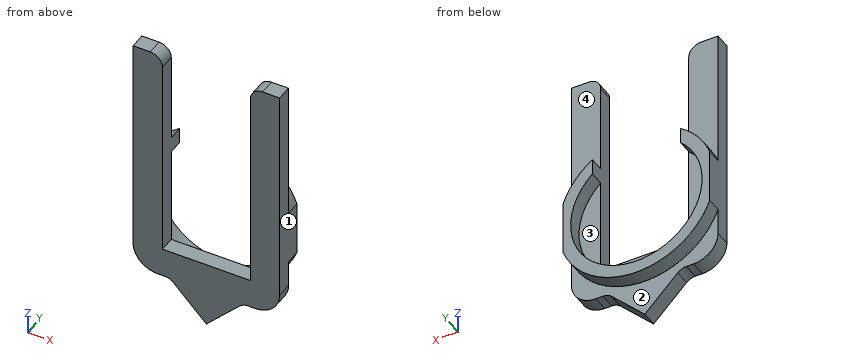
```python
from build123d import *

# Parameters (mm, degrees)
BOSS_EXTRUDE1_DEPTH = 3.2
BOSS_EXTRUDE2_DEPTH = 3
FILLET1_R           = 5
FILLET2_R           = 2.5


with BuildPart() as part:
    # Sketch1 → Boss-Extrude1 (new body)
    with BuildSketch(Plane(origin=(0, 0, 0), x_dir=(1, 0, 0), z_dir=(0, 1, 0))):
        Polygon((-15, -25), (-9, -25), (-9, 19), (9, 19), (9, -25), (15, -25), (15, 25), (7.5, 25), (0, 32.5), (-7.5, 25), (-15, 25), align=None)
    extrude(amount=BOSS_EXTRUDE1_DEPTH)

    # Sketch2 → Boss-Extrude2 (add)
    with BuildSketch(Plane(origin=(0, 3.2, 0), x_dir=(1, 0, 0), z_dir=(0, 1, 0))):
        with BuildLine():
            Line((-9, -4.228756555), (-9, -1))
            ThreePointArc((-9, -1), (0, 22.453624047), (9, -1))
            Line((9, -1), (9, -4.228756555))
            ThreePointArc((9, -4.228756555), (12.596535252, -0.865459931), (15, 3.432235637))
            Line((15, 3.432235637), (15, 14.567764363))
            ThreePointArc((15, 14.567764363), (0, 25), (-15, 14.567764363))
            Line((-15, 14.567764363), (-15, 3.432235637))
            ThreePointArc((-15, 3.432235637), (-12.596535252, -0.865459931), (-9, -4.228756555))
        make_face()
    extrude(amount=BOSS_EXTRUDE2_DEPTH)

    # Fillet1
    fillet1_edges = [part.edges().sort_by_distance(p)[0] for p in [
        (15, 1.6, -25),
        (-15, 1.6, -25),
    ]]
    fillet(fillet1_edges, radius=FILLET1_R)

    # Fillet2
    fillet2_edges = [part.edges().sort_by_distance(p)[0] for p in [
        (-7.5, 1.6, -25),
        (7.5, 1.6, -25),
        (9, 1.6, 25),
        (-9, 1.6, 25),
    ]]
    fillet(fillet2_edges, radius=FILLET2_R)


solid = part.part
```
Geometry: final body of the model. Coordinates: model frame, mm. Face numbers are marked on the shaded views. A direction names the side the tool comes from. Round coordinates to 2 decimals unless told otherwise and drop trailing zeros. Order: outer loops, then holes, each group sorted by start corner. A loop starts at its lowest first (then second) coordinate and runs counter-clockwise, first axis right, second up. Notation, with made-up numbers: (24.25, 62.5) -> (69.25, 62.5) arc R21 cw to (69.25, 89.5) -> close; hole circle Ø9 at (52.25, -38). An arc over 180 degrees is marked (long way). Use one line per item in the form item = value. Start each with the question number.
1. Cut plane B-B (y = 1.5). Return the cut outline in (x, z), then the cut area to 3 significant figures.
2. Cut plane C-C (x = -6). Return the cut outline in (y, z).
3. Cut plane D-D (z = 13). Return the cut outline in (x, y).
4. Line query: probe 1 along X at (y, z) = (5, -9); probe 2 along X at (y, z) = (2.75, -2); probe 3 along Z at (x, y) = (0, 3.9). Output: solid intervals per line, ascending.
5. Pin query (flat end, axial travel): pin 1 Ø1.2 at (x, y) = (9, 1) entering from -Z; pin 2 Ø1 at (x, z) = (1.5, -20.5) entering from +Y; pin 3 Ø1.6 at (x, y) = (4, 2.5) entering from +Z. Return the tip coordinate at first contact, or that it passes through.
6. Reachability of the marked faces 1 and 2 from +Z, -Z, +X, -X, +Y, -Y: full face, straight path, thin tool, end or side. Return the list, or none.
7. Draft query along Z for the marked faces 3 and 4. Return one class per face: pulls with the +Z half, pulls with the -Z half, needs draft (parallel to the pull), parting line crosses it, or undercut.
8. Cut plane A-A (z = -9). Return the cut outline in (x, y).
Solution:
q1.outline = (-15, -20) arc R5 ccw to (-10, -25) -> (-8.54, -25) arc R2.5 cw to (-6.77, -25.73) -> (0, -32.5) -> (6.77, -25.73) arc R2.5 cw to (8.54, -25) -> (10, -25) arc R5 ccw to (15, -20) -> (15, 25) -> (11.5, 25) arc R2.5 ccw to (9, 22.5) -> (9, -19) -> (-9, -19) -> (-9, 22.5) arc R2.5 ccw to (-11.5, 25) -> (-15, 25) -> close
q1.area = 751 mm^2
q2.outline = (0, -26.5) -> (3.2, -26.5) -> (3.2, -23.83) -> (6.2, -23.83) -> (6.2, -21.04) -> (3.2, -21.04) -> (3.2, -19) -> (0, -19) -> close
q3.outline = (-15, 0) -> (-9, 0) -> (-9, 3.2) -> (-15, 3.2) -> close; (9, 0) -> (15, 0) -> (15, 3.2) -> (9, 3.2) -> close
q4.probe_1 = -15 to -13.45, 13.45 to 15
q4.probe_2 = -15 to -9, 9 to 15
q4.probe_3 = -25 to -22.45
q5.pin_1 = -25
q5.pin_2 = 3.2
q5.pin_3 = -19
q6.face_1 = +Z, -Z, +X, +Y, -Y
q6.face_2 = -Z, +Y
q7.face_3 = undercut
q7.face_4 = needs draft
q8.outline = (-15, 0) -> (-9, 0) -> (-9, 3.2) -> (-13.45, 3.2) -> (-13.45, 6.2) -> (-15, 6.2) -> close; (9, 0) -> (15, 0) -> (15, 6.2) -> (13.45, 6.2) -> (13.45, 3.2) -> (9, 3.2) -> close
